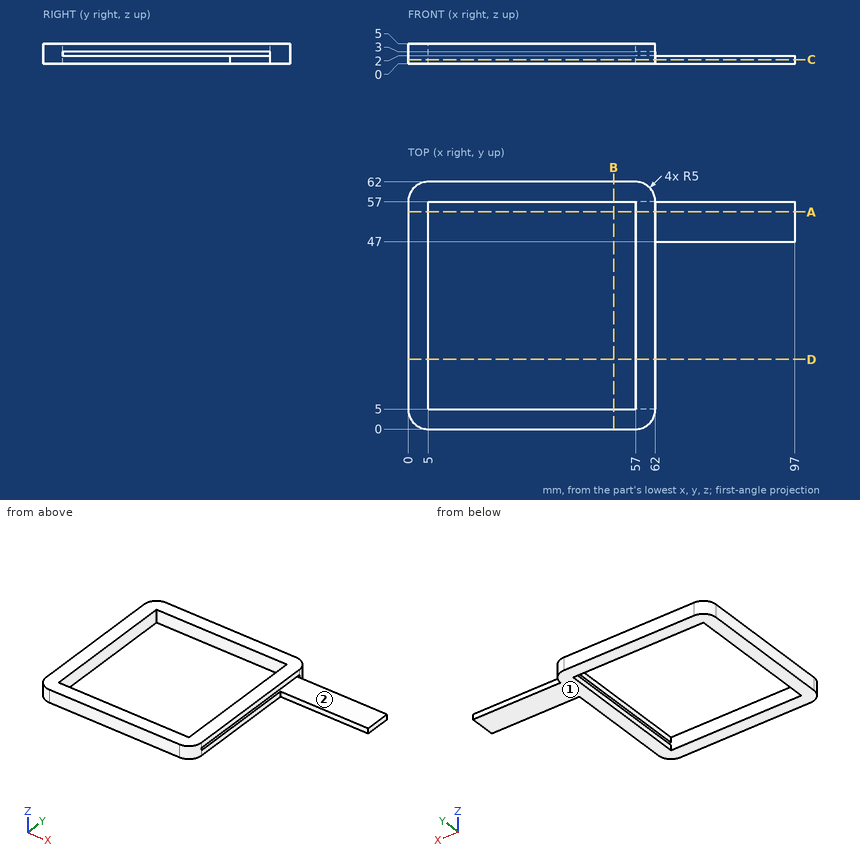
Design review of the part shown in the three views and the two pictorial views. Dimensions are in mm from the part's minimum x, y and z. Round coordinates to 2 decimals unless told otherwise and drop trailing zeros. Order: outer loops, then holes, each group sorted by start corner. A loop starts at its lowest first (then second) coordinate and runs counter-clockwise, first axis right, second up. Notation, with made-up numbers: (83, -12) -> (142, -12) arc R33 ccw to (142, 25) -> close; hole circle Ø3 at (9.25, 50.25). An arc over 180 degrees is marked (long way). Write item = value, one per line. Start each with the question number.
1) Insertion check: pin 1 (2 mm diameter, centred on x = 70, y = 51.5, fed in from +Z); pin 2 (0.6 mm diameter, centred on x = 76.5, z = 1, fed in from +Y); pin 3 (2 mm diameter, centred on y = 33, z = 1.5, fed in from +X). Each pin has a flat end and moves straight along its axis. Give the tip position at first contact, or say it passes through.
2) Take a section at C-C on z = 1.1. State the section outline as (x, y) points, plus the area to 3 significant figures.
3) Take a section at B-B on x = 51.5. State the section outline as (y, z) points, plus the area to 3 significant figures.
4) The part is to be moulded in two halves that separate along Y. For the marked faces 1 and 2, say which applies: +Y half, -Y half, draft (parallel to the pull), parting line (faces both ways), or undercut.
5) To check wall thickness, follow line 1 (Y direction, x = 12.5, z = 2); line 2 (X direction, y = 15, z = 2.3). State the ranges of each line that lie inside material, in increasing order. Write a range as from..to.
6) Take a section at D-D on y = 17.5. State the section outline as (x, z) points, plus the area to 3 significant figures.
7) Take a section at A-A on y = 54.5. State the section outline as (x, z) points.
Verdict:
q1.pin_1 = 2
q1.pin_2 = 57
q1.pin_3 = 62
q2.outline = (0, 5) arc R5 ccw to (5, 0) -> (57, 0) arc R5 ccw to (62, 5) -> (62, 47) -> (97, 47) -> (97, 57) -> (62, 57) arc R5 ccw to (57, 62) -> (5, 62) arc R5 ccw to (0, 57) -> close; hole (5, 5) -> (57, 5) -> (57, 57) -> (5, 57) -> close
q2.area = 1,470 mm2
q3.outline = (0, 0) -> (5, 0) -> (5, 5) -> (0, 5) -> close; (57, 0) -> (62, 0) -> (62, 5) -> (57, 5) -> close
q3.area = 50.0 mm2
q4.face_1 = draft
q4.face_2 = undercut
q5.line_1 = 0..5, 57..62
q5.line_2 = 0..5
q6.outline = (0, 0) -> (5, 0) -> (5, 5) -> (0, 5) -> close; (57, 0) -> (62, 0) -> (62, 2) -> (57, 2) -> close; (57, 3) -> (62, 3) -> (62, 5) -> (57, 5) -> close
q6.area = 45.0 mm2
q7.outline = (0, 0) -> (5, 0) -> (5, 5) -> (0, 5) -> close; (57, 0) -> (97, 0) -> (97, 2) -> (57, 2) -> close; (57, 3) -> (62, 3) -> (62, 5) -> (57, 5) -> close
